The model under review builds one solid part; all positions refer to its coordinate system, in mm. A direction names the side the tool comes from. Round coordinates to 2 decimals unless told otherwise and drop trailing zeros. Loops run counter-clockwise (first coordinate to the right, second up) from the corner with the lowest first, then second, coordinate; pieces in that order, holes last. Notation, with made-up numbers: (49.25, 68) -> (102.25, 68) arc R23 ccw to (102.25, 102) -> close; hole circle Ø11 at (-35, 82.5). An arc over 180 degrees is marked (long way). Write each question's results on one line, items separated by ' | '. Start each with the question number.
Item 1: We need section C-C (x = -16.5). Give the boundary of the cut face in (y, z).
Item 2: For L1, parallel to Z at x = -25, y = 25; L2, parallel to X at y = 24.7, z = -14; L3, parallel to X at y = 33, z = -6.5, list the stretches that pass through material, from the lowest coordinate up. Write a range as from..to.
Item 3: Mouldability with a two-part tool opening along Y and no side actions: class faces 1 (the cylindrical face through (-25.954, 25.502, 10.2)), 2 (the flat face through (-23.9, 27.5, 10.9)), 3 (the cylindrical face through (16.3, 39.2, 39.5)) as pulls with the +Y half, pulls with the -Y half, needs draft (parallel to the pull), parting line crosses it, or undercut.
Item 4: We need section D-D (z = 2). Give the boundary of the cut face in (x, y), and give its area (3 significant figures).
Item 5: We need section B-B (z = 35). Give the boundary of the cut face in (x, y), and give its area (3 significant figures).
Item 6: We need section A-A (y = 25.75). Give the boundary of the cut face in (x, z).
Item 7: Clearance check with flat-ended pins moving along their axes: pin 1 Ø4 at (x, y) = (4.5, 30) entering from +Z; pin 2 Ø8 at (y, z) = (37, 9.5) entering from -X; pin 3 Ø10 at (y, z) = (39.5, 32) entering from +X. State where each tip first meets the part, or that it passes through.
Item 8: Tool access review of faces 4 (the flat face through (-21, 36, 10)), 5 (the cylindrical face through (25, 25, -13)), 6 (the flat face through (-15.082, 28, -12)), 7 (the flat face through (23, 27.5, 11)), 8 (the flat face through (-17, 40, 37)): name each direction out of +Z, -Z, +X, -X, +Y, -Y from which nothing blocks a thin tool from reaching the whole face with its end or side.
Autodesk Inventor part; units mm, degrees
ref_plane "YZ Plane" through (0, 0, 0) normal (1, 0, 0) x (0, 1, 0)
ref_plane "XZ Plane" through (0, 0, 0) normal (0, 1, 0) x (-1, 0, 0)
ref_plane "XY Plane" through (0, 0, 0) normal (0, 0, 1) x (1, 0, 0)
sketch "Sketch1" plane through (0, 0, 0) normal (0, 1, 0) x (-1, 0, 0)
  circle A0 centre (0, 0) radius 11 construction
  circle A1 centre (0, 0) radius 3.75
  circle A2 centre (0, 0) radius 7.875 construction
  line L0 (16.292, 0) -> (-19, 0) construction
  line L1 (0, 21) -> (0, -27.3544) construction
  line L2 (0, -21) -> (21, -21)
  line L3 (0, -21) -> (-21, -21)
  line L4 (0, 0) -> (21, -21) construction
  circle A3 centre (5.5685, -5.5685) radius 0.75
  circle A4 centre (-5.5685, -5.5685) radius 0.75
  circle A5 centre (5.5685, 5.5685) radius 0.75
  circle A6 centre (-5.5685, 5.5685) radius 0.75
  line L5 (-28, -21) -> (-21, -21)
  line L6 (28, -21) -> (21, -21)
  circle A7 centre (25, -14) radius 1
  circle A8 centre (-25, -14) radius 1
  line L7 (-28, 42) -> (28, 42)
  line L8 (28, -21) -> (28, 42)
  line L9 (21, -21) -> (21, 42)
  line L10 (-21, -21) -> (-21, 42)
  line L11 (-28, -21) -> (-28, 42)
  line L12 (28, 10.5) -> (-28, 10.5) construction
  circle A9 centre (25, 35) radius 1
  circle A10 centre (-25, 35) radius 1
  circle A11 centre (25, 10.5) radius 1
  circle A12 centre (-25, 10.5) radius 1
  circle A13 centre (5.5685, 5.5685) radius 1.5
  circle A14 centre (5.5685, -5.5685) radius 1.5
  circle A15 centre (-5.5685, 5.5685) radius 1.5
  circle A16 centre (-5.5685, -5.5685) radius 1.5
  dimension "d8" = 15.75
  dimension "d2" = 7.5
  dimension "d4" = 22
  dimension "d17" = 21
  dimension "d26" = 1.5
  dimension "d38" = 63
  dimension "d39" = 21
  dimension "d40" = 2
  dimension "d41" = 2
  dimension "d53" = 3
  dimension "d97" = 7
  dimension "d98" = 3
  dimension "d99" = 3
extrude "Extrusion9" add sketch "Sketch1" along normal blind 45 contours A1 | L3 L10 L7 L9 L2 | A3 | A4 | A5 | A6 | A13 | A14 | A15 | A16
extrude "Extrusion10" add sketch "Sketch1" along normal blind 27.5 contours L9 L7 L8 L6 | L5 L11 L7 L10
extrude "Extrusion11" cut sketch "Sketch1" along normal blind 17.5 contours L9 L7 L8 L6 | L5 L11 L7 L10
extrude "Extrusion13" cut sketch "Sketch1" along normal blind 6 contours A1 | A3 | A4 | A5 | A6 | A13 | A14 | A15 | A16
extrude "Extrusion15" add sketch "Sketch1" along normal blind 3.5 contours A13 | A14 | A15 | A16
sketch "Sketch5" plane through (-21, 45, 42) normal (0, 0, 1) x (1, 0, 0)
  line L0 (0, -45) -> (42, -45) construction
  line L1 (0, -17.5) -> (0, 0) construction
  line L2 (42, -45) -> (0, -45) construction
  line L3 (0, -45) -> (0, 0) construction
  line L4 (0, 0) -> (42, 0) construction
  line L5 (42, 0) -> (42, -45) construction
  line L6 (42, 0) -> (0, -45) construction
  line L7 (0, 0) -> (42, 0) construction
  line L8 (0, 0) -> (42, -45) construction
  circle A0 centre (21, -22.5) radius 18.5
  line L9 (10.2856, -7.4185) -> (31.7144, -7.4185)
  line L10 (5.9185, -11.7856) -> (5.9185, -33.2144)
  line L11 (36.0815, -11.7856) -> (36.0815, -33.2144)
  circle A1 centre (21, -22.5) radius 13.5 construction
  line L12 (34.0815, -9.4185) -> (7.9185, -35.5815) construction
  line L13 (21, -45) -> (21, 0) construction
  line L14 (7.9185, -9.4185) -> (34.0815, -35.5815) construction
  line L15 (7.9185, -9.4185) -> (34.0815, -9.4185) construction
  line L16 (7.9185, -9.4185) -> (7.9185, -35.5815) construction
  line L17 (34.0815, -35.5815) -> (34.0815, -9.4185) construction
  circle A2 centre (4.5, -40.1786) radius 1
  circle A3 centre (37.5, -40.1786) radius 1
  circle A4 centre (4.5, -4.8214) radius 1
  circle A5 centre (37.5, -4.8214) radius 1
  line L18 (50, -22.5352) -> (50, -23.5001)
  line L19 (50, -22.5352) -> (-3.9988, -22.4696) construction
  line L20 (50, -23.5001) -> (42, -23.5001)
  line L21 (42, -23.5001) -> (39.473, -23.5)
  line L22 (39.473, -23.5) -> (36.0815, -23.5)
  line L23 (36.0815, -23.5) -> (21, -23.5)
  line L24 (50, -23.5001) -> (50, -45)
  line L25 (50, -45) -> (21, -45)
  line L26 (-8, -23.5001) -> (0, -23.5001)
  line L27 (0, -23.5001) -> (2.527, -23.5)
  line L28 (2.527, -23.5) -> (5.9185, -23.5)
  line L29 (5.9185, -23.5) -> (21, -23.5)
  line L30 (-8, -23.5001) -> (-8, -45)
  line L31 (-8, -45) -> (21, -45)
  line L32 (-8, -22.4648) -> (-8, -23.5001)
  line L33 (50, -22.5352) -> (50.0023, -21.5703)
  line L34 (50.0023, -21.5703) -> (42.0024, -21.5509)
  line L35 (42.0024, -21.5509) -> (39.4753, -21.5449)
  line L36 (39.4753, -21.5449) -> (36.0839, -21.5367)
  line L37 (36.0839, -21.5367) -> (21.0024, -21.5)
  line L38 (50.0023, -21.5703) -> (50.0546, -0.0706)
  line L39 (50.0546, -0.0706) -> (21.0547, -0.0001)
  line L40 (-7.9452, 0.0704) -> (21.0547, -0.0001)
  line L41 (-7.9975, -21.4294) -> (-7.9452, 0.0704)
  line L42 (-7.9975, -21.4294) -> (0.0025, -21.4488)
  line L43 (0.0025, -21.4488) -> (2.5295, -21.4551)
  line L44 (2.5295, -21.4551) -> (5.921, -21.4633)
  line L45 (5.921, -21.4633) -> (21.0024, -21.5)
  line L46 (-8, -22.4648) -> (-7.9975, -21.4294)
  point P0 (39.5, -22.5225)
  dimension "d58" = 37
  dimension "d70" = 27
  dimension "d73" = 2
  dimension "d74" = 45
  dimension "d75" = 2
  dimension "d76" = 2
  dimension "d77" = 42
  dimension "d79" = 2
  dimension "d80" = 4.5
  dimension "d89" = 1
  dimension "d90" = 1
  dimension "d93" = 29
extrude "Extrusion16" cut sketch "Sketch5" against normal blind 62 contours L11 L37 L45 L44 L10 A0 L9 | A0 L10 L29 L23 L11 | L23 L29 L10 L44 L45 L37 L11
extrude "Extrusion18" cut sketch "Sketch5" against normal blind 46 contours A0 L22 L11 L37 L36 | L36 L37 L11 A0 | A0 L11 L22 | L9 A0 | A0 L28 L10 | A0 L44 L10 L28 | L10 L44 A0
extrude "Extrusion19" cut sketch "Sketch5" against normal blind 5 contours A2 | A3 | A4 | A5
extrude "Extrusion23" cut sketch "Sketch5" against normal blind 70 contours A0 L22 L11 L37 L36 | A0 L35 L34 L33 L18 L20 L21 | L21 L20 L24 L25 L31 L30 L26 L27 A0 | A0 L11 L22 | A0 L10 L29 L23 L11 | L23 L29 L10 L44 L45 L37 L11 | A0 L28 L10 | L27 L26 L32 L46 L42 L43 A0 | A0 L44 L10 L28 | A2 | A3
fillet "Fillet1" radius 1 20 edges at (-28, 27.5, 10.5) (-24.5, 27.5, 42) (-28, 25.5341, 42) (-21, 27.5, 10.5) (-24.5, 27.5, -21) (-28, 25.5341, -21) (-21, 36.25, -21) (-21, 45, 10.5) (0, 45, -21) (21, 36.25, -21) (24.5, 27.5, -21) (28, 25.466, -21) (21, 27.5, 10.5) (28, 27.5, 10.5) (21, 36.25, 42) (0, 45, 42) (21, 45, 10.5) (-21, 36.25, 42) (24.5, 27.5, 42) (28, 25.466, 42)
equation "\"d41\" = d40"
properties part number "engine_sleeve_down"
Here are the results:
1) outline: (23.54, -21) -> (44, -21) arc R1 ccw to (45, -20) -> (45, 41) arc R1 ccw to (44, 42) -> (41.18, 42) -> (41.18, 37) -> (39.18, 37) -> (39.18, 42) -> (30.87, 42) -> (30.87, -4) -> (23.54, -4) -> close
2) L1: z = -21..-15, -13..9.5, 11.5..34, 36..42 | L2: x = -28..-26, -24..-15.08, 15.08..24, 26..28 | L3: x = -21..-15.08, 15.08..21
3) face 1: needs draft | face 2: pulls with the +Y half | face 3: undercut
4) outline: (-28, 23.57) -> (-21, 23.55) -> (-18.47, 23.54) arc R18.5 cw to (18.48, 23.46) -> (21, 23.45) -> (28, 23.43) -> (28, 26.5) arc R1 ccw to (27, 27.5) -> (22, 27.5) arc R1 cw to (21, 28.5) -> (21, 44) arc R1 ccw to (20, 45) -> (-20, 45) arc R1 ccw to (-21, 44) -> (-21, 28.5) arc R1 cw to (-22, 27.5) -> (-27, 27.5) arc R1 ccw to (-28, 26.5) -> close | area: 458 mm2
5) outline: (-28, 23.57) -> (-26, 23.56) -> (-26, 27.5) -> (-27, 27.5) arc R1 ccw to (-28, 26.5) -> close; (-24, 23.56) -> (-21, 23.55) -> (-18.47, 23.54) arc R18.5 cw to (18.48, 23.46) -> (21, 23.45) -> (24, 23.44) -> (24, 27.5) -> (22, 27.5) arc R1 cw to (21, 28.5) -> (21, 44) arc R1 ccw to (20, 45) -> (-20, 45) arc R1 ccw to (-21, 44) -> (-21, 28.5) arc R1 cw to (-22, 27.5) -> (-24, 27.5) -> close; (26, 23.44) -> (28, 23.43) -> (28, 26.5) arc R1 ccw to (27, 27.5) -> (26, 27.5) -> close | area: 442 mm2
6) outline: (-28, -20) arc R1 ccw to (-27, -21) -> (27, -21) arc R1 ccw to (28, -20) -> (28, 41) arc R1 ccw to (27, 42) -> (18.21, 42) -> (18.21, -4) -> (15.08, -4) -> (15.08, -20) -> (-15.08, -20) -> (-15.08, -4) -> (-18.21, -4) -> (-18.21, 42) -> (-27, 42) arc R1 ccw to (-28, 41) -> close; hole circle Ø2 at (-25, -14); hole circle Ø2 at (-25, 10.5); hole circle Ø2 at (-25, 35); hole circle Ø2 at (25, -14); hole circle Ø2 at (25, 10.5); hole circle Ø2 at (25, 35)
7) pin 1: stops at z = -20 | pin 2: stops at x = -21 | pin 3: stops at x = 21
8) face 4: +Z, -Z, -X, +Y | face 5: +Y, -Y | face 6: +Z, -Y | face 7: +Z, -Z, +X, +Y | face 8: +Z
